Work out the finished part from the listing and answer in its coordinate system (mm). Give positions to 0.01 mm unless a question says otherwise; leave off trailing zeros. Order: outer loops, then holes, each group sorted by start corner. A loop starts at its lowest first (then second) coordinate and runs counter-clockwise, first axis right, second up.
```python
from build123d import *

# Parameters (mm, degrees)
F0_R     = 13.5
F1_DEPTH = 7
F2_D     = 1.2
F3_R     = 3


with BuildPart() as f1:
    # F0 (on Top) → F1 (new body)
    with BuildSketch(Plane.XY):
        Circle(F0_R)
    extrude(amount=F1_DEPTH)

    # F2 (through all)
    with Locations(Plane(origin=(0, 0, 0), x_dir=(1, 0, 0), z_dir=(0, 0, -1))):
        with Locations((0, 0)):
            Hole(F2_D / 2)

    # F3
    f3_edges = [f1.edges().sort_by_distance(p)[0] for p in [
        (-13.5, 0, 0),
        (-13.5, 0, 7),
    ]]
    fillet(f3_edges, radius=F3_R)


solid = f1.part
```
1. The part is cut by section C-C (z = 1.25). Write down the section's boundary in (x, y).
Findings below:
outline: circle Ø25.87 at (0, 0); hole circle Ø1.2 at (0, 0)
2. The mould has two halves that part along X. Classify faces 1 (the face through (0, -2, 7)), 2 (the face through (-2.93, -13.18, 3.49)), 3 (the face through (-0.323, -0.506, 3.549)): pulls with the +X half, pulls with the -X half, needs draft (parallel to the pull), parting line crosses it, or undercut.
Findings below:
face 1: needs draft
face 2: parting line crosses it
face 3: undercut
3. Straight lines are drawn through the part: probe 1 along Y at (x, z) = (0, 3.5); probe 2 along Y at (x, z) = (0, 5); probe 3 along X at (y, z) = (11, 4). For each, find the intervals that lie inside material, in ascending order.
Findings below:
probe 1: y = -13.5 to -0.6, 0.6 to 13.5
probe 2: y = -13.33 to -0.6, 0.6 to 13.33
probe 3: x = -7.83 to 7.83
4. Given P1, Ø1, axis at y = -10, z = 6, coming from the +X side; P2, Ø3, axis at x = -3.5, z = 3, coming from the -Y side; P3, Ø2, axis at y = 7, z = 1, coming from the -X side; P4, Ø0.7, axis at x = 0, y = 0, coming from the -Z side, each flat-ended and moving along its own axis, determine where each tip first touches the part or whether it passes through.
Findings below:
P1: stops at x = 8.73
P2: stops at y = -13.35
P3: stops at x = -11.61
P4: passes through
5. The part is cut by section A-A (y = 0). Write down the section's boundary in (x, z), then the cut area to 3 significant figures.
Findings below:
outline: (-13.5, 3) arc R3 ccw to (-10.5, 0) - (-0.6, 0) - (-0.6, 7) - (-10.5, 7) arc R3 ccw to (-13.5, 4) - close; (0.6, 0) - (10.5, 0) arc R3 ccw to (13.5, 3) - (13.5, 4) arc R3 ccw to (10.5, 7) - (0.6, 7) - close
area: 173 mm2
